Job drawing, mm, ordinate dimensions from the low corner. One solid piece. A direction names the side the tool comes from. Round coordinates to 2 decimals unless told otherwise and drop trailing zeros. Loops run counter-clockwise (first coordinate to the right, second up) from the corner with the lowest first, then second, coordinate; pieces in that order, holes last.
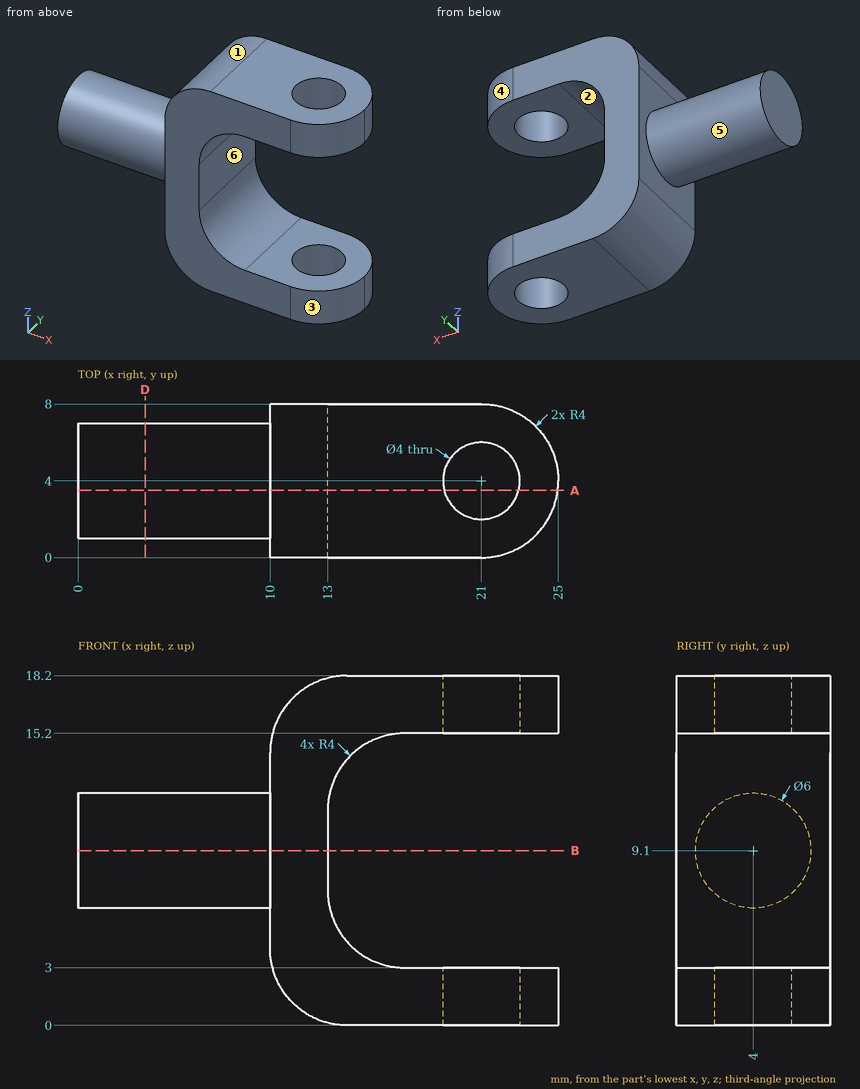
Item 1: Flat gauge pins, fed straight in: P1, Ø3.5, axis at y = 3, z = 9, coming from the +X side; P2, Ø2.5, axis at x = 21, y = 4, coming from the -Z side. Where does each tip first touch, or does it go through?
Answers follow:
P1: stops at x = 13
P2: passes through
Item 2: Two-plate mould, pull along Z, no slides. Class the marked faces 1, 2 and 3: released by +Z, released by -Z, zero draft, split by the parting line, or undercut.
Answers follow:
face 1: released by +Z
face 2: undercut
face 3: zero draft
Item 3: Cut at A-A, the plane y = 3.5. Give the cut face in (x, z), plus the area to 3 significant figures.
Answers follow:
outline: (0, 6.14) - (10, 6.14) - (10, 4) arc R4 ccw to (14, 0) - (19.06, 0) - (19.06, 3) - (17, 3) arc R4 cw to (13, 7) - (13, 11.2) arc R4 cw to (17, 15.2) - (19.06, 15.2) - (19.06, 18.2) - (14, 18.2) arc R4 ccw to (10, 14.2) - (10, 12.06) - (0, 12.06) - close; (22.94, 0) - (24.97, 0) - (24.97, 3) - (22.94, 3) - close; (22.94, 15.2) - (24.97, 15.2) - (24.97, 18.2) - (22.94, 18.2) - close
area: 162 mm2
Item 4: 3-axis set-ups, long thin cutter, end or side, ignore diameter. For the marked faces 4, 5 and 6: which of +Z, -Z, +X, -X, +Y, -Y reach the whole face in a straight line?
Answers follow:
face 4: +Z, -Z, +X, +Y
face 5: -X
face 6: +X, +Y, -Y
Item 5: Cut at D-D, the plane x = 3.5. Give the cut face in (y, z).
Answers follow:
outline: circle Ø6 at (4, 9.1)
Item 6: Probe line 1 (Z direction, x = 23, y = 5.5); line 2 (Y direction, x = 21, z = 16.2); line 3 (X direction, y = 0.5, z = 7.5). List the from-to ranges inside material, lowest first.
Answers follow:
line 1: z = 0 to 3, 15.2 to 18.2
line 2: y = 0 to 2, 6 to 8
line 3: x = 10 to 13
Item 7: Cut at B-B, the plane z = 9.1. Give the cut face in (x, y), plus the area to 3 significant figures.
Answers follow:
outline: (0, 1) - (10, 1) - (10, 0) - (13, 0) - (13, 8) - (10, 8) - (10, 7) - (0, 7) - close
area: 84.0 mm2
